```python
from build123d import *

# Parameters (mm, degrees)
SKETCH002_W  = 2
SKETCH002_H  = 25
PAD001_DEPTH = 15
PAD_DEPTH    = 7.5


with BuildPart() as pad001:
    # Sketch002 → Pad001 (new body, symmetric)
    with BuildSketch(Plane.XZ):
        with Locations((0, -13.5)):
            Rectangle(SKETCH002_W, SKETCH002_H)
    extrude(amount=PAD001_DEPTH, both=True)


with BuildPart() as pad:
    # Sketch001 → Pad (new body, symmetric)
    with BuildSketch(Plane.XZ):
        Polygon((8, -26.856406), (0, -13), (-8, -26.856406), align=None)
    extrude(amount=PAD_DEPTH, both=True)


with BuildPart() as cut001:
    # Sketch → Revolution (revolve)
    with BuildSketch(Plane.XZ):
        Polygon((0, 4), (8.5, 4), (10, 2.5), (10, 0), (5.1, 0), (5.1, -13.058023), (5.5, -13.750843), (5.20287, -18), (0, -18), align=None)
    revolve(axis=Axis((0, 0, 0), (0, 0, 1)))

    # Cut: cut Pad
    add(pad.part, mode=Mode.SUBTRACT)

    # Cut001: cut Pad001
    add(pad001.part, mode=Mode.SUBTRACT)


solid = cut001.part
```
The listing builds one solid part. Answer for the finished solid, in the listing's coordinates (mm). A direction names the side the tool comes from. Round coordinates to 2 decimals unless told otherwise and drop trailing zeros. Write each loop counter-clockwise with the first axis right and the second up, starting at its lowest first coordinate (ties: lowest second). Pieces come first, ordered by that corner, then holes. Notation, with made-up numbers: (-32.75, -7) -> (4.25, -7) arc R21 cw to (4.25, 20) -> close; hole circle Ø2 at (47.25, 61.5). An arc over 180 degrees is marked (long way). Use CSV: the item, a comma, the result in double quotes. Start each with the question number.
(1) Which of the six approach directions +Z, -Z, +X, -X, +Y, -Y give full straight-line access (tool end or side, diameter ignored) to faces 4 (the face through (5.213, -0.101, -13.255)), 5 (the face through (-5.213, 0.101, -13.255)), 6 (the face through (0, 0, -1))?
(2) Section C-C on z = -5.25 is taken. Give the vertices of the cut face in (x, y), then the cut area to 3 significant figures.
(3) The mould has two halves that part along X. Classify faces 1 (the face through (-1.93, -0.07, -16.34)), 2 (the face through (0, 0, 4)), 3 (the face through (-5.35, 0.1, -15.91)): released by +X, released by -X, zero draft, split by the parting line, or undercut.
(4) Section B-B on x = 0 is taken. Give the vertices of the cut face in (y, z).
(5) Consider L1, parallel to Z at x = 5.75, y = 0.5; L2, parallel to X at y = -2.25, z = -8.5; L3, parallel to X at y = 1, z = -5.5. Determine where each line is inside the solid, lowest interval first. Write a range as from..to.
(6) Section A-A on y = 0 is taken. Give the vertices of the cut face in (x, z), then the cut area to 3 significant figures.
(7) Each of these flat-tipped pins is pushed along its axis until it touches: pin 1 (3 mm diameter, centred on y = -1, z = -10.5, fed in from +X); pin 2 (10 mm diameter, centred on y = -7, z = 0.5, fed in from -X); pin 3 (10 mm diameter, centred on x = -7.5, z = -14, fed in from -Y). Where does it stop, or does it pass through?
A:
1,face 4,"+X"
1,face 5,"-X"
1,face 6,"-Z, +Y, -Y"
2,outline,"(-1, -5) -> (-1, 5) arc R5.1 ccw to start; (1, -5) arc R5.1 ccw to (1, 5) -> close"
2,area,"61.4 mm²"
3,face 1,"undercut"
3,face 2,"zero draft"
3,face 3,"released by -X"
4,outline,"(-10, 0) -> (-5.1, 0) -> (-5.1, -1) -> (5.1, -1) -> (5.1, 0) -> (10, 0) -> (10, 2.5) -> (8.5, 4) -> (-8.5, 4) -> (-10, 2.5) -> close"
5,L1,"z = 0..4"
5,L2,"x = -4.58..-1, 1..4.58"
5,L3,"x = -5..-1, 1..5"
6,outline,"(-10, 0) -> (-5.1, 0) -> (-5.1, -13.06) -> (-5.5, -13.75) -> (-5.2, -18) -> (-2.89, -18) -> (-1, -14.73) -> (-1, -1) -> (1, -1) -> (1, -14.73) -> (2.89, -18) -> (5.2, -18) -> (5.5, -13.75) -> (5.1, -13.06) -> (5.1, 0) -> (10, 0) -> (10, 2.5) -> (8.5, 4) -> (-8.5, 4) -> (-10, 2.5) -> close"
6,area,"224 mm²"
7,pin 1,"stops at x = 5.1"
7,pin 2,"stops at x = -9.8"
7,pin 3,"stops at y = -4.9"
